from build123d import *

# Parameters (mm, degrees)
SKETCH1_W           = 40
SKETCH1_H           = 40
SKETCH1_W_2         = 34
SKETCH1_H_2         = 34
BOSS_EXTRUDE1_DEPTH = 70
SKETCH2_W           = 34
SKETCH2_H           = 3
BOSS_EXTRUDE2_DEPTH = 37
CUT_EXTRUDE1_DEPTH  = 37
SKETCH4_R           = 8.5
SKETCH4_R_2         = 7.5
BOSS_EXTRUDE3_DEPTH = 2
SKETCH6_R           = 7.5
BOSS_EXTRUDE4_DEPTH = 10
FILLET2_R           = 1.5
FILLET3_R           = 1.5
FILLET4_R           = 1.5
FILLET5_R           = 1.5


with BuildPart() as part:
    # Sketch1 → Boss-Extrude1 (new body)
    with BuildSketch(Plane.XY):
        with Locations((-20, 20)):
            Rectangle(SKETCH1_W, SKETCH1_H)
        with Locations((-20, 20)):
            Rectangle(SKETCH1_W_2, SKETCH1_H_2, mode=Mode.SUBTRACT)
    extrude(amount=BOSS_EXTRUDE1_DEPTH)

    # Sketch2 → Boss-Extrude2 (add)
    with BuildSketch(Plane(origin=(0, 37, 0), x_dir=(-1, 0, 0), z_dir=(0, -1, 0))):
        with Locations((20, -68.5)):
            Rectangle(SKETCH2_W, SKETCH2_H)
    extrude(amount=BOSS_EXTRUDE2_DEPTH)

    # Sketch3 → Cut-Extrude1 (cut)
    with BuildSketch(Plane(origin=(0, 40, 0), x_dir=(1, 0, 0), z_dir=(0, 1, 0))):
        with BuildLine():
            ThreePointArc((-12.5, -15), (-14.696699141, -9.696699141), (-20, -7.5))
            Line((-20, -7.5), (-20, -15))
            Line((-20, -15), (-12.5, -15))
        make_face()
        with BuildLine():
            Line((-20, -15), (-20, -7.5))
            ThreePointArc((-20, -7.5), (-25.303300859, -9.696699141), (-27.5, -15))
            Line((-27.5, -15), (-20, -15))
        make_face()
        with BuildLine():
            Line((-12.5, -15), (-20, -15))
            Line((-20, -15), (-20, -22.5))
            ThreePointArc((-20, -22.5), (-14.696699141, -20.303300859), (-12.5, -15))
        make_face()
        with BuildLine():
            Line((-20, -22.5), (-20, -15))
            Line((-20, -15), (-27.5, -15))
            ThreePointArc((-27.5, -15), (-25.303300859, -20.303300859), (-20, -22.5))
        make_face()
        with BuildLine():
            ThreePointArc((-12.5, -55), (-14.696699141, -49.696699141), (-20, -47.5))
            Line((-20, -47.5), (-20, -55))
            Line((-20, -55), (-12.5, -55))
        make_face()
        with BuildLine():
            Line((-20, -55), (-20, -47.5))
            ThreePointArc((-20, -47.5), (-25.303300859, -49.696699141), (-27.5, -55))
            Line((-27.5, -55), (-20, -55))
        make_face()
        with BuildLine():
            Line((-12.5, -55), (-20, -55))
            Line((-20, -55), (-20, -62.5))
            ThreePointArc((-20, -62.5), (-14.696699141, -60.303300859), (-12.5, -55))
        make_face()
        with BuildLine():
            Line((-20, -62.5), (-20, -55))
            Line((-20, -55), (-27.5, -55))
            ThreePointArc((-27.5, -55), (-25.303300859, -60.303300859), (-20, -62.5))
        make_face()
    extrude(amount=-CUT_EXTRUDE1_DEPTH, mode=Mode.SUBTRACT)

    # Sketch4 → Boss-Extrude3 (add)
    with BuildSketch(Plane(origin=(0, 37, 0), x_dir=(-1, 0, 0), z_dir=(0, -1, 0))):
        with Locations((20, -15)):
            Circle(SKETCH4_R)
        with Locations((20, -15)):
            Circle(SKETCH4_R_2, mode=Mode.SUBTRACT)
        with Locations((20, -55)):
            Circle(SKETCH4_R)
        with Locations((20, -55)):
            Circle(SKETCH4_R_2, mode=Mode.SUBTRACT)
    extrude(amount=BOSS_EXTRUDE3_DEPTH)

    # Sketch6 → Boss-Extrude4 (add)
    with BuildSketch(Plane(origin=(0, 3, 0), x_dir=(1, 0, 0), z_dir=(0, 1, 0))):
        with Locations((-20, -15)):
            Circle(SKETCH6_R)
        with Locations((-20, -55)):
            Circle(SKETCH6_R)
    extrude(amount=-BOSS_EXTRUDE4_DEPTH)

    # Fillet2
    fillet2_edges = [part.edges().sort_by_distance(p)[0] for p in [
        (-27.5, -7, 55),
    ]]
    fillet(fillet2_edges, radius=FILLET2_R)

    # Fillet3
    fillet3_edges = [part.edges().sort_by_distance(p)[0] for p in [
        (-27.5, -7, 15),
    ]]
    fillet(fillet3_edges, radius=FILLET3_R)

    # Fillet4
    fillet4_edges = [part.edges().sort_by_distance(p)[0] for p in [
        (-27.5, 0, 15),
    ]]
    fillet(fillet4_edges, radius=FILLET4_R)

    # Fillet5
    fillet5_edges = [part.edges().sort_by_distance(p)[0] for p in [
        (-27.5, 0, 55),
    ]]
    fillet(fillet5_edges, radius=FILLET5_R)


solid = part.part
For this review, take the finished solid that the model builds, in its own axes (mm). A direction names the side the tool comes from. Round coordinates to 2 decimals unless told otherwise and drop trailing zeros. Order: outer loops, then holes, each group sorted by start corner. A loop starts at its lowest first (then second) coordinate and runs counter-clockwise, first axis right, second up. Notation, with made-up numbers: M 58,17 L 111,17 A21 cw 111,40 Z; hole C -26,65 d2. An arc over 180 degrees is marked long. Write each question's results on one line, items separated by ' | '. Start each with the question number.
1. Add section A-A (y = 8). State the section outline as (x, z) points, then the cut area to 3 significant figures.
2. Draft analysis for pull direction X (two halves, no side actions). For faces 4 (the face through (-20, 35, 63)), 5 (the face through (-20, -7, 15)), 6 (the face through (-27.493, -3.472, 54.67)), state which applies: pulls with the +X half, pulls with the -X half, needs draft (parallel to the pull), parting line crosses it, or undercut.
3. Add section B-B (y = -2.5). State the section outline as (x, z) points, then the cut area to 3 significant figures.
4. To check wall thickness, follow L1, parallel to Z at x = -20, y = 36.25; L2, parallel to X at y = 36.1, z = 55; L3, parallel to X at y = 4, z = 28. State the ranges of each line that lie inside material, in increasing order. Write a range as [from, to].
5. Clearance check with a flat-ended pin moving along its axis: pin 1 Ø12 at (x, z) = (-20, 15) entering from +Y. State where the tip first meets the part, or that it passes through.
6. Tool access review of faces 1 (the face through (-37, 20, 33)), 2 (the face through (-13.255, 36.014, 60.172)), 3 (the face through (-27.493, -3.472, 14.67)): name each direction out of +Z, -Z, +X, -X, +Y, -Y from which nothing blocks a thin tool from reaching the whole face with its end or side.
7. Add section C-C (x = -24.5). State how many separate pieces and enclosed holes the cut face has, then the cut area to 3 significant figures.
Output values:
1) outline: M -40,0 L -37,0 L -37,67 L -3,67 L -3,0 L 0,0 L 0,70 L -40,70 Z | area: 522 mm^2
2) face 4: undercut | face 5: needs draft | face 6: parting line crosses it
3) outline: C -20,15 d15; C -20,55 d15 | area: 353 mm^2
4) L1: [6.5, 7.5], [22.5, 23.5], [46.5, 47.5], [62.5, 63.5], [67, 70] | L2: [-40, -37], [-28.5, -27.5], [-12.5, -11.5], [-3, 0] | L3: [-40, -37], [-3, 0]
5) pin 1: y = 3
6) face 1: -Z | face 2: none | face 3: -Y
7) separate pieces: 3 | enclosed holes: 0 | area: 628 mm^2
